Check sheet for the modelled part. Datum: model origin and axes. Units: mm. A direction names the side the tool comes from. Coordinates: 2 decimals unless noted, no trailing zeros. Loops run counter-clockwise (first coordinate to the right, second up) from the corner with the lowest first, then second, coordinate; pieces in that order, holes last.
```python
from build123d import *

# Parameters (mm, degrees)
SKETCH1_W            = 152.4
SKETCH1_H            = 101.6
BOSS_EXTRUDE1_DEPTH  = 6.35
BOSS_EXTRUDE2_DEPTH  = 6.35
SKETCH5_R            = 12.7
BOSS_EXTRUDE3_DEPTH  = 1.27
BOSS_EXTRUDE4_DEPTH  = 2.38125
RIB1_REACH           = 212.988
SKETCH7_WALL_W       = 480.772618864
SKETCH7_WALL_H       = 2.54
SKETCH8_R            = 6.35
CUT_EXTRUDE1_DEPTH   = 207.100301795
SKETCH9_R            = 4.7625
CUT_EXTRUDE2_DEPTH   = 195.376393886
LPATTERN1_COUNT      = 2
LPATTERN1_PITCH      = 127
LPATTERN1_COUNT_DIR2 = 2
LPATTERN1_PITCH_DIR2 = 76.2


with BuildPart() as part:
    # Sketch1 → Boss-Extrude1 (new body)
    with BuildSketch(Plane.XY):
        Rectangle(SKETCH1_W, SKETCH1_H)
    extrude(amount=BOSS_EXTRUDE1_DEPTH)

    # Sketch4 → Boss-Extrude2 (add)
    with BuildSketch(Plane(origin=(0, 19.05, 0), x_dir=(1, 0, 0), z_dir=(0, 1, 0))):
        with BuildLine():
            Line((63.5, -6.35), (18.312580006, -163.998991669))
            ThreePointArc((18.312580006, -163.998991669), (0, -177.8), (-18.312580006, -163.998991669))
            Line((-18.312580006, -163.998991669), (-63.5, -6.35))
            Line((-63.5, -6.35), (63.5, -6.35))
        make_face()
    extrude(amount=-BOSS_EXTRUDE2_DEPTH)

    # Sketch5 → Boss-Extrude3 (add)
    with BuildSketch(Plane(origin=(0, 19.05, 0), x_dir=(1, 0, 0), z_dir=(0, 1, 0))):
        with Locations((0, -158.75)):
            Circle(SKETCH5_R)
    extrude(amount=BOSS_EXTRUDE3_DEPTH)

    # Sketch6 → Boss-Extrude4 (add, symmetric)
    with BuildSketch(Plane(origin=(0, 0, 0), x_dir=(0, 0, -1), z_dir=(1, 0, 0))):
        Polygon((-6.35, -38.1), (-146.05, 12.7), (-6.35, 12.7), align=None)
    extrude(amount=BOSS_EXTRUDE4_DEPTH, both=True)

    # Sketch7 wall → Rib1 (add, up to next)
    with BuildSketch(Plane(origin=(25.4, 0, 31.75), x_dir=(0, -0.4472135955, -0.894427191), z_dir=(0, 0.894427191, -0.4472135955)), mode=Mode.PRIVATE) as rib1_sk1:
        Rectangle(SKETCH7_WALL_W, SKETCH7_WALL_H)
    rib1_tool1 = extrude(rib1_sk1.sketch, amount=RIB1_REACH, mode=Mode.PRIVATE) - part.part
    rib1 = rib1_tool1.solids().sort_by_distance((25.4, 0, 31.75))[0]
    add(rib1)

    # Mirror1: Rib1 across plane
    add(rib1.mirror(Plane(origin=(0, 0, 0), x_dir=(0, 0, 1), z_dir=(1, 0, 0))))

    # Sketch8 → Cut-Extrude1 (cut, through all)
    with BuildSketch(Plane(origin=(0, 20.32, 0), x_dir=(1, 0, 0), z_dir=(0, 1, 0))):
        with Locations(Location((0, -158.75, 0), (0, 0, 180))):
            Circle(SKETCH8_R)
    extrude(amount=-CUT_EXTRUDE1_DEPTH, mode=Mode.SUBTRACT)

    # Sketch9 → Cut-Extrude2 (cut, symmetric)
    with BuildSketch(Plane.XY.offset(6.35)):
        with Locations((-63.5, 38.1)):
            Circle(SKETCH9_R)
    cut_extrude2 = extrude(amount=CUT_EXTRUDE2_DEPTH, both=True, mode=Mode.SUBTRACT)

    # LPattern1: Cut-Extrude2 2 × 2
    with Locations(*[(i * LPATTERN1_PITCH, -j * LPATTERN1_PITCH_DIR2, 0) for i in range(LPATTERN1_COUNT) for j in range(LPATTERN1_COUNT_DIR2) if (i, j) != (0, 0)]):
        add(cut_extrude2, mode=Mode.SUBTRACT)


solid = part.part
```
1) Scan lines: line 1 (Y direction, x = 63, z = 4); line 2 (Z direction, x = -12.5, y = 1); line 3 (Y direction, x = 5, z = 62). Record each from-to range of solid material in increasing order.
Answer sheet:
line 1: y = -50.8 to -42.84, -33.36 to 33.36, 42.84 to 50.8
line 2: z = 0 to 6.35
line 3: y = 12.7 to 19.05
2) Set-up check for faces 4 (the flat face through (25.38, 0.18, 32.11)), 5 (the flat face through (-25.38, 0.18, 32.11)), 6 (the flat face through (2.381, -7, 60)), 7 (the flat face through (-6, 20.32, 156)), 8 (the flat face through (-1, 1, 0)): record each of +Z, -Z, +X, -X, +Y, -Y from which the full face is reachable in a straight line by a thin tool's end or side.
Answer sheet:
face 4: +Z, +X, -Y
face 5: +Z, -X, -Y
face 6: +Z, -Y
face 7: +Z, +X, -X, +Y
face 8: -Z, +X, -X, +Y, -Y
3) Depth check by flat-ended pin: pin 1 (20.5 mm diameter, centred on x = -3.5, z = 162, fed in from +Y); pin 2 (6 mm diameter, centred on x = -35, z = 91.5, fed in from +Y); pin 3 (12.5 mm diameter, centred on y = 1, z = 39.5, fed in from +X); pin 4 (1 mm diameter, centred on x = -58, y = 38, fed in from -Z). Enter the tip coordinate at first touch or a pass-through.
Answer sheet:
pin 1: stops at y = 20.32
pin 2: stops at y = 19.05
pin 3: stops at x = 26.67
pin 4: stops at z = 0
4) Section check D-D on z = 25. Enter the section's corners in (x, y) (3 decimals), plus the area to 3 significant figures.
Answer sheet:
outline: (-58.154, 12.7) - (-26.67, 12.7) - (-26.67, -3.375) - (-24.13, -3.375) - (-24.13, 12.7) - (-2.381, 12.7) - (-2.381, -31.318) - (2.381, -31.318) - (2.381, 12.7) - (24.13, 12.7) - (24.13, -3.375) - (26.67, -3.375) - (26.67, 12.7) - (58.154, 12.7) - (58.154, 19.05) - (-58.154, 19.05) - close
area: 1,030 mm2
5) Section check A-A on y = 16. Enter the section's corners in (x, z), plus the area to 3 significant figures.
Answer sheet:
outline: (-76.2, 0) - (76.2, 0) - (76.2, 6.35) - (63.5, 6.35) - (18.31, 164) arc R19.05 ccw to (-18.31, 164) - (-63.5, 6.35) - (-76.2, 6.35) - close; hole circle Ø12.7 at (0, 158.75)
area: 14,100 mm2
6) Section check B-B on x = 0. Enter the section's corners in (y, z), plus the area to 3 significant figures.
Answer sheet:
outline: (-50.8, 0) - (50.8, 0) - (50.8, 6.35) - (19.05, 6.35) - (19.05, 146.05) - (20.32, 146.05) - (20.32, 152.4) - (12.7, 152.4) - (12.7, 146.05) - (-38.1, 6.35) - (-50.8, 6.35) - close; (12.7, 165.1) - (20.32, 165.1) - (20.32, 171.45) - (19.05, 171.45) - (19.05, 177.8) - (12.7, 177.8) - close
area: 5,220 mm2
7) Mould release check, pull along Z, two halves, no side actions. Record for faces 1 (the cylindrical face through (-68.258, -37.891, 3.219)), 2 (the cylindrical face through (0.344, 15.919, 177.797)), 3 (the cylindrical face through (-2.75, 19.68, 171.15)): +Z half, -Z half, draft (parallel to the pull), parting line (faces both ways), or undercut.
Answer sheet:
face 1: draft
face 2: +Z half
face 3: undercut
8) Section check C-C on y = 38.1. Enter the section's corners in (x, z).
Answer sheet:
outline: (-76.2, 0) - (-68.26, 0) - (-68.26, 6.35) - (-76.2, 6.35) - close; (-58.74, 0) - (58.74, 0) - (58.74, 6.35) - (-58.74, 6.35) - close; (68.26, 0) - (76.2, 0) - (76.2, 6.35) - (68.26, 6.35) - close
